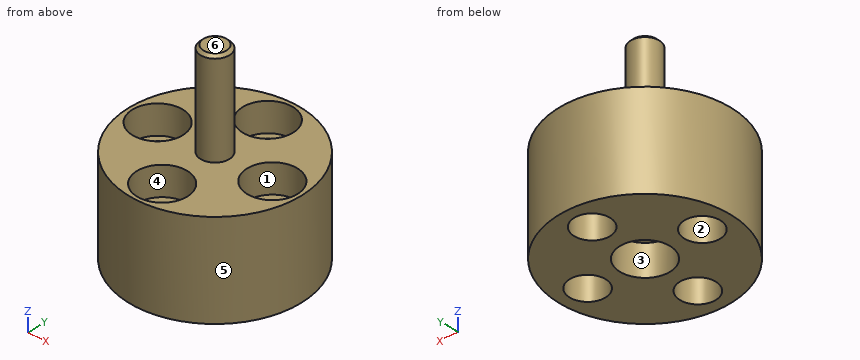
```python
from build123d import *

# Parameters (mm, degrees)
SKETCH1_R                                        = 19.05
SKETCH1_R_2                                      = 5
SKETCH1_R_3                                      = 3.96875
BOSS_EXTRUDE1_DEPTH                              = 21
BOSS_EXTRUDE2_START                              = -14.142
SKETCH3_R                                        = 5
BOSS_EXTRUDE2_DEPTH                              = 14.142
SKETCH4_R                                        = 3.175
BOSS_EXTRUDE3_DEPTH                              = 21
CHAMFER1_SIZE                                    = 0.635
CBORE_FOR_1_4_SOCKET_HEAD_CAP_SCREW1_D           = 6.7564
CBORE_FOR_1_4_SOCKET_HEAD_CAP_SCREW1_CBORE_D     = 11.1125
CBORE_FOR_1_4_SOCKET_HEAD_CAP_SCREW1_CBORE_DEPTH = 6.35


with BuildPart() as part:
    # Sketch1 → Boss-Extrude1 (new body)
    with BuildSketch(Plane.XY):
        Circle(SKETCH1_R)
        Circle(SKETCH1_R_2, mode=Mode.SUBTRACT)
        with Locations((0, 12.7)):
            Circle(SKETCH1_R_3, mode=Mode.SUBTRACT)
        with Locations((12.7, 0)):
            Circle(SKETCH1_R_3, mode=Mode.SUBTRACT)
        with Locations((0, -12.7)):
            Circle(SKETCH1_R_3, mode=Mode.SUBTRACT)
        with Locations((-12.7, 0)):
            Circle(SKETCH1_R_3, mode=Mode.SUBTRACT)
    extrude(amount=BOSS_EXTRUDE1_DEPTH)

    # Sketch3 → Boss-Extrude2 (add)
    with BuildSketch(Plane(origin=(0, 0, 6.858), x_dir=(-1, 0, 0), z_dir=(0, 0, -1)).offset(BOSS_EXTRUDE2_START)):
        Circle(SKETCH3_R)
    extrude(amount=BOSS_EXTRUDE2_DEPTH)

    # Sketch4 → Boss-Extrude3 (add)
    with BuildSketch(Plane.XY.offset(21)):
        Circle(SKETCH4_R)
    extrude(amount=BOSS_EXTRUDE3_DEPTH)

    # Chamfer1
    chamfer1_edges = [part.edges().sort_by_distance(p)[0] for p in [
        (-3.175, 0, 42),
    ]]
    chamfer(chamfer1_edges, length=CHAMFER1_SIZE)

    # CBORE for 1/4 Socket Head Cap Screw1 (through all)
    with Locations(Plane.XY.offset(21)):
        with Locations((0, 12.7), (12.7, 0), (0, -12.7), (-12.7, 0)):
            CounterBoreHole(CBORE_FOR_1_4_SOCKET_HEAD_CAP_SCREW1_D / 2, CBORE_FOR_1_4_SOCKET_HEAD_CAP_SCREW1_CBORE_D / 2, CBORE_FOR_1_4_SOCKET_HEAD_CAP_SCREW1_CBORE_DEPTH)

    # Sketch7 → CBORE for 1/4 Socket Head Cap Screw2 (revolve, cut)
    with BuildSketch(Plane.YZ):
        Polygon((0, 0), (0, 2.055227343), (3.3782, 0.0254), (3.3782, 6.858), (5.55625, 6.858), (5.55625, 0), align=None)
    revolve(axis=Axis((0, 0, -6.35), (0, 0, 1)), mode=Mode.SUBTRACT)


solid = part.part
```
Work out the finished part from the listing and answer in its coordinate system (mm). Face numbers are marked on the shaded views. A direction names the side the tool comes from. Coordinates: 2 decimals unless noted, no trailing zeros. Write each loop counter-clockwise with the first axis right and the second up, starting at its lowest first coordinate (ties: lowest second). Pieces come first, ordered by that corner, then holes. Notation, with made-up numbers: (30, -26.75) - (80, -26.75) arc R22 ccw to (80, -10.75) - close; hole circle Ø2 at (63.5, 18.5). An arc over 180 degrees is marked (long way). Answer as a JSON object with one key per item and string values.
Q1. Find section C-C (z = 9). Write down the section's boundary in (x, y), plus the area to 3 significant figures.
Results list:
{"outline": "circle Ø38.1 at (0, 0); hole circle Ø7.94 at (-12.7, 0); hole circle Ø7.94 at (0, -12.7); hole circle Ø7.94 at (0, 12.7); hole circle Ø7.94 at (12.7, 0)", "area": "942 mm^2"}
Q2. Given pin 1 Ø14.5 at (x, y) = (12.7, 0) entering from +Z; pin 2 Ø5 at (x, z) = (-6.5, 15) entering from -Y; pin 3 Ø10.5 at (x, y) = (0, 12.7) entering from +Z, each flat-ended and moving along its own axis, determine where each tip first touches the part or whether it passes through.
Results list:
{"pin 1": "stops at z = 21", "pin 2": "stops at y = -18.63", "pin 3": "stops at z = 14.65"}
Q3. Which of the six approach directions +Z, -Z, +X, -X, +Y, -Y give full straight-line access (tool end or side, diameter ignored) to the marked faces 1 and 2?
Results list:
{"face 1": "+Z", "face 2": "+Z, -Z"}
Q4. Find section D-D (y = -15). Write down the section's boundary in (x, z), plus the area to 3 significant figures.
Results list:
{"outline": "(-11.74, 0) - (-3.23, 0) - (-3.23, 14.65) - (-5.06, 14.65) - (-5.06, 21) - (-11.74, 21) - close; (3.23, 0) - (11.74, 0) - (11.74, 21) - (5.06, 21) - (5.06, 14.65) - (3.23, 14.65) - close", "area": "334 mm^2"}
Q5. Consider L1, parallel to Y at x = 0, z = 11.25; L2, parallel to Y at x = 0, z = 3; L3, parallel to Y at x = 0, z = 18. Determine where each line is inside the solid, lowest interval first. Write a range as from..to.
Results list:
{"L1": "y = -19.05..-16.67, -8.73..8.73, 16.67..19.05", "L2": "y = -19.05..-16.67, -8.73..-5.56, 5.56..8.73, 16.67..19.05", "L3": "y = -19.05..-18.26, -7.14..7.14, 18.26..19.05"}
Q6. Find section A-A (x = 0). State how many separate pieces and enclosed holes the cut face has, plus the area to 3 significant figures.
Results list:
{"separate pieces": "3", "enclosed holes": "0", "area": "483 mm^2"}
Q7. For a pull along Y with two mould halves and no side action, classify the marked faces 3, 4, 5 and 6 as pulls with the +Y half, pulls with the -Y half, needs draft (parallel to the pull), parting line crosses it, or undercut.
Results list:
{"face 3": "undercut", "face 4": "undercut", "face 5": "parting line crosses it", "face 6": "needs draft"}
